from build123d import *

# Parameters (mm, degrees)
F0_R     = 17.5
F1_DEPTH = 11
F2_SIZE  = 0.5
F3_R     = 7.5
F4_DEPTH = 40.7
F5_SIZE  = 0.5


with BuildPart() as f1:
    # F0 (on Top) → F1 (new body)
    with BuildSketch(Plane.XY):
        Circle(F0_R)
    extrude(amount=F1_DEPTH)

    # F2
    f2_edges = [f1.edges().sort_by_distance(p)[0] for p in [
        (-17.5, 0, 11),
        (-17.5, 0, 0),
    ]]
    chamfer(f2_edges, length=F2_SIZE)

    # F3 (on face) → F4 (cut)
    with BuildSketch(Plane.XY.offset(11)):
        Circle(F3_R)
    extrude(amount=-F4_DEPTH, mode=Mode.SUBTRACT)

    # F5
    f5_edges = [f1.edges().sort_by_distance(p)[0] for p in [
        (-7.5, 0, 11),
        (-7.5, 0, 0),
    ]]
    chamfer(f5_edges, length=F5_SIZE)


solid = f1.part
The listing builds one solid part. Answer for the finished solid, in the listing's coordinates (mm). Give positions to 0.01 mm unless a question says otherwise; leave off trailing zeros. Write each loop counter-clockwise with the first axis right and the second up, starting at its lowest first coordinate (ties: lowest second). Pieces come first, ordered by that corner, then holes.
1) Find the intervals of material crossed by L1, parallel to Y at x = 0, z = 3.25; L2, parallel to Y at x = -5, z = 5.75; L3, parallel to X at y = 4, z = 8.25, in increasing order.
2) Given P1, Ø2, axis at y = 12.5, z = 10, coming from the -X side; P2, Ø4, axis at x = -9, z = 7.5, coming from the +Y side; P3, Ø3, axis at y = -9, z = 6.5, coming from the -X side, each flat-ended and moving along its own axis, determine where each tip first touches the part or whether it passes through.
3) For a pull along Y with two mould halves and no side action, classify faces 1 (the face through (-13.887, -10.648, 5.43)), 2 (the face through (7.3, 4, 0)), 3 (the face through (-7.493, 0.33, 5.57)) as pulls with the +Y half, pulls with the -Y half, needs draft (parallel to the pull), parting line crosses it, or undercut.
4) Section C-C (z = 8.75) is taken. Write down the section's boundary in (x, y), and give its area (3 significant figures).
5) Section A-A (y = 0) is taken. Write down the section's boundary in (x, z).
Response:
1. L1: y = -17.5 to -7.5, 7.5 to 17.5
1. L2: y = -16.77 to -5.59, 5.59 to 16.77
1. L3: x = -17.04 to -6.34, 6.34 to 17.04
2. P1: stops at x = -13.19
2. P2: stops at y = 16.04
2. P3: stops at x = -15.81
3. face 1: parting line crosses it
3. face 2: needs draft
3. face 3: undercut
4. outline: circle Ø35 at (0, 0); hole circle Ø15 at (0, 0)
4. area: 785 mm2
5. outline: (-17.5, 0.5) - (-17, 0) - (-8, 0) - (-7.5, 0.5) - (-7.5, 10.5) - (-8, 11) - (-17, 11) - (-17.5, 10.5) - close; (7.5, 0.5) - (8, 0) - (17, 0) - (17.5, 0.5) - (17.5, 10.5) - (17, 11) - (8, 11) - (7.5, 10.5) - close
